```python
from build123d import *

# Parameters (mm, degrees)
ESQUISSE2_R             = 2.5
ESQUISSE2_R_2           = 7.5
ESQUISSE2_R_3           = 1.5
BOSS_EXTRU_5_DEPTH      = 5
ESQUISSE3_W             = 49
ESQUISSE3_H             = 12.5
ENL_V_MAT_EXTRU_1_DEPTH = 1
ESQUISSE4_R             = 2
ENL_V_MAT_EXTRU_2_DEPTH = 130.272649712


with BuildPart() as part:
    # Esquisse2 → Boss.-Extru.5 (new body)
    with BuildSketch(Plane(origin=(0, 0, 0), x_dir=(1, 0, 0), z_dir=(0, 1, 0))):
        with BuildLine():
            Line((-75.214465703, -26.391441925), (-75.214465703, -31.391441925))
            Line((-75.214465703, -31.391441925), (-15.214465703, -31.391441925))
            Line((-15.214465703, -31.391441925), (-15.214465703, -26.391441925))
            Line((-15.214465703, -26.391441925), (24.785534297, -26.391441925))
            Line((24.785534297, -26.391441925), (24.785534297, -31.391441925))
            Line((24.785534297, -31.391441925), (51.321432682, -31.391441925))
            ThreePointArc((51.321432682, -31.391441925), (54.785534297, -33.391441925), (58.249635912, -31.391441925))
            Line((58.249635912, -31.391441925), (84.785534297, -31.391441925))
            Line((84.785534297, -31.391441925), (84.785534297, -26.391441925))
            Line((84.785534297, -26.391441925), (119.785534297, -26.391441925))
            Line((119.785534297, -26.391441925), (119.785534297, -8.891441925))
            Line((119.785534297, -8.891441925), (124.785534297, -8.891441925))
            Line((124.785534297, -8.891441925), (124.785534297, 11.108558075))
            Line((124.785534297, 11.108558075), (119.785534297, 11.108558075))
            Line((119.785534297, 11.108558075), (119.785534297, 28.608558075))
            Line((119.785534297, 28.608558075), (84.785534297, 28.608558075))
            Line((84.785534297, 28.608558075), (84.785534297, 23.608558075))
            Line((84.785534297, 23.608558075), (24.785534297, 23.608558075))
            Line((24.785534297, 23.608558075), (24.785534297, 28.608558075))
            Line((24.785534297, 28.608558075), (-15.214465703, 28.608558075))
            Line((-15.214465703, 28.608558075), (-15.214465703, 23.608558075))
            Line((-15.214465703, 23.608558075), (-75.214465703, 23.608558075))
            Line((-75.214465703, 23.608558075), (-75.214465703, 28.608558075))
            Line((-75.214465703, 28.608558075), (-110.214465703, 28.608558075))
            Line((-110.214465703, 28.608558075), (-110.214465703, 11.108558075))
            Line((-110.214465703, 11.108558075), (-115.214465703, 11.108558075))
            Line((-115.214465703, 11.108558075), (-115.214465703, -8.891441925))
            Line((-115.214465703, -8.891441925), (-110.214465703, -8.891441925))
            Line((-110.214465703, -8.891441925), (-110.214465703, -26.391441925))
            Line((-110.214465703, -26.391441925), (-75.214465703, -26.391441925))
        make_face()
        with Locations(Location((54.785534297, -29.391441925, 0), (0, 0, 270))):
            Circle(ESQUISSE2_R, mode=Mode.SUBTRACT)
        with Locations(Location((-90.214465703, -3.891441925, 0), (0, 0, 270))):
            Circle(ESQUISSE2_R_2, mode=Mode.SUBTRACT)
        with Locations(Location((99.785534297, -3.891441925, 0), (0, 0, 270))):
            Circle(ESQUISSE2_R_2, mode=Mode.SUBTRACT)
        with Locations(Location((-105.214465703, 3.608558075, 0), (0, 0, 270))):
            Circle(ESQUISSE2_R_3, mode=Mode.SUBTRACT)
        with Locations(Location((-75.214465703, 3.608558075, 0), (0, 0, 270))):
            Circle(ESQUISSE2_R_3, mode=Mode.SUBTRACT)
        with Locations(Location((-96.714465703, 16.108558075, 0), (0, 0, 270))):
            Circle(ESQUISSE2_R_3, mode=Mode.SUBTRACT)
        with Locations(Location((-83.714465703, 16.108558075, 0), (0, 0, 270))):
            Circle(ESQUISSE2_R_3, mode=Mode.SUBTRACT)
        with Locations(Location((84.785534297, 3.608558075, 0), (0, 0, 270))):
            Circle(ESQUISSE2_R_3, mode=Mode.SUBTRACT)
        with Locations(Location((114.785534297, 3.608558075, 0), (0, 0, 270))):
            Circle(ESQUISSE2_R_3, mode=Mode.SUBTRACT)
        with Locations(Location((93.285534297, 16.108558075, 0), (0, 0, 270))):
            Circle(ESQUISSE2_R_3, mode=Mode.SUBTRACT)
        with Locations(Location((106.285534297, 16.108558075, 0), (0, 0, 270))):
            Circle(ESQUISSE2_R_3, mode=Mode.SUBTRACT)
    extrude(amount=BOSS_EXTRU_5_DEPTH)

    # Esquisse3 → Enlèv. mat.-Extru.1 (cut)
    with BuildSketch(Plane(origin=(0, 5, 0), x_dir=(1, 0, 0), z_dir=(0, 1, 0))):
        with Locations((54.785534297, 17.358558075)):
            Rectangle(ESQUISSE3_W, ESQUISSE3_H)
        with Locations((-45.214465703, 17.358558075)):
            Rectangle(ESQUISSE3_W, ESQUISSE3_H)
    extrude(amount=-ENL_V_MAT_EXTRU_1_DEPTH, mode=Mode.SUBTRACT)

    # Esquisse4 → Enlèv. mat.-Extru.2 (cut, through all)
    with BuildSketch(Plane(origin=(0, 5, 0), x_dir=(1, 0, 0), z_dir=(0, 1, 0))):
        with Locations(Location((72.285534297, 17.108558075, 0), (0, 0, 270))):
            Circle(ESQUISSE4_R)
        with Locations(Location((37.285534297, 17.108558075, 0), (0, 0, 90))):
            Circle(ESQUISSE4_R)
        with Locations(Location((-27.714465703, 17.108558075, 0), (0, 0, 270))):
            Circle(ESQUISSE4_R)
        with Locations(Location((-62.714465703, 17.108558075, 0), (0, 0, 90))):
            Circle(ESQUISSE4_R)
    extrude(amount=-ENL_V_MAT_EXTRU_2_DEPTH, mode=Mode.SUBTRACT)


solid = part.part
```
Geometry check sheet. Reference: the model listing, model coordinates, mm. A direction names the side the tool comes from. Give positions to 0.01 mm unless a question says otherwise; leave off trailing zeros. Loops run counter-clockwise (first coordinate to the right, second up) from the corner with the lowest first, then second, coordinate; pieces in that order, holes last. Notation, with made-up numbers: M -28,-32.75 L 0,-32.75 A22 ccw 0,-19.75 Z; hole C 56.25,19.25 d9. An arc over 180 degrees is marked long. Answer as CSV lines item,"result".
Item 1: Depth check by flat-ended pin: P1, Ø2.5, axis at x = 106.29, z = -16.11, coming from the +Y side; P2, Ø5, axis at x = 72.29, z = -17.11, coming from the +Y side; P3, Ø1.5, axis at x = 35, y = 1.5, coming from the +Z side; P4, Ø1.5, axis at x = -99, y = 2.5, coming from the +Z side. Enter the tip coordinate at first touch or a pass-through.
Values:
P1,"passes through"
P2,"stops at y = 4"
P3,"stops at z = 31.39"
P4,"stops at z = 26.39"
Item 2: Cross-section at C-C on y = 2.4. Count the separate pieces of the cut face and the enclosed holes in it, and give its area (3 significant figures).
Values:
separate pieces,"1"
enclosed holes,"15"
area,"12,400 mm²"
Item 3: Cross-section at B-B on z = 14. Record the cut outline in (x, y), and give its area (3 significant figures).
Values:
outline,"M -110.21,0 L 119.79,0 L 119.79,5 L -110.21,5 Z"
area,"1,150 mm²"
Item 4: Cross-section at A-A on x = 61.5. Record the cut outline in (y, z), and give its area (4 significant figures).
Values:
outline,"M 0,-23.61 L 4,-23.61 L 4,-11.11 L 5,-11.11 L 5,31.39 L 0,31.39 Z"
area,"262.5 mm²"
Item 5: Access from +Z, -Z, +X, -X, +Y, -Y to the whole of each face (thin tool, end or side, straight path). Record for faces 4 (the flat face through (-92, 2, -28.609)), 5 (the flat face through (122, 2, -11.109)), 6 (the flat face through (71, 2, 31.391)), 7 (the flat face through (-15.214, 2, -26)), 8 (the flat face through (-110.214, 2, -20)).
Values:
face 4,"-Z, +X, -X, +Y, -Y"
face 5,"-Z, +X, +Y, -Y"
face 6,"+Z, +X, +Y, -Y"
face 7,"-Z, +Y, -Y"
face 8,"-Z, -X, +Y, -Y"
Item 6: Cross-section at D-D on x = 6.5. Record the cut outline in (y, z), and give its area (3 significant figures).
Values:
outline,"M 0,-28.61 L 5,-28.61 L 5,26.39 L 0,26.39 Z"
area,"275 mm²"
Item 7: Release check for a two-part mould opening along X. For faces 1 (the cylindrical face through (-82.778, 2.465, 2.915)), 2 (the flat face through (84.786, 2, 29)), 3 (the flat face through (3, 0, 2)) record: pulls with the +X half, pulls with the -X half, needs draft (parallel to the pull), parting line crosses it, or undercut.
Values:
face 1,"undercut"
face 2,"pulls with the +X half"
face 3,"needs draft"
Item 8: Material ranges on line 1 (X direction, y = 3.9, z = 8); line 2 (X direction, y = 2.55, z = -2); line 3 (Z direction, x = 59.5, y = 3.5), recorded low to high.
Values:
line 1,"x = -115.21 to -96.49, -83.94 to 93.51, 106.06 to 124.79"
line 2,"x = -115.21 to -94.86, -85.57 to 95.14, 104.43 to 124.79"
line 3,"z = -23.61 to 31.39"
